from build123d import *

# Parameters (mm, degrees)
BOSS_EXTRUDE1_DEPTH                         = 300
CBORE_FOR_M3_BUTTON_HEAD_SCREW1_D           = 3.4
CBORE_FOR_M3_BUTTON_HEAD_SCREW1_CBORE_D     = 6.7
CBORE_FOR_M3_BUTTON_HEAD_SCREW1_CBORE_DEPTH = 6.15
LPATTERN1_COUNT                             = 12
LPATTERN1_PITCH                             = 25


with BuildPart() as part:
    # Sketch1 → Boss-Extrude1 (new body)
    with BuildSketch(Plane(origin=(0, 0, 0), x_dir=(0, 0, -1), z_dir=(1, 0, 0))):
        with BuildLine():
            Line((0, 5.5), (0, 0))
            Line((0, 0), (12, 0))
            Line((12, 0), (12, 5.5))
            ThreePointArc((12, 5.5), (11.5, 6), (12, 6.5))
            Line((12, 6.5), (12, 8))
            Line((12, 8), (0, 8))
            Line((0, 8), (0, 6.5))
            ThreePointArc((0, 6.5), (0.5, 6), (0, 5.5))
        make_face()
    extrude(amount=-BOSS_EXTRUDE1_DEPTH)

    # CBORE for M3 Button Head Screw1 (through all)
    with Locations(Plane(origin=(0, 8, 0), x_dir=(1, 0, 0), z_dir=(0, 1, 0))):
        with Locations((-288, 6)):
            cbore_for_m3_button_head_screw1 = CounterBoreHole(CBORE_FOR_M3_BUTTON_HEAD_SCREW1_D / 2, CBORE_FOR_M3_BUTTON_HEAD_SCREW1_CBORE_D / 2, CBORE_FOR_M3_BUTTON_HEAD_SCREW1_CBORE_DEPTH)

    # LPattern1: CBORE for M3 Button Head Screw1 ×12
    with Locations(*[(i * LPATTERN1_PITCH, 0, 0) for i in range(1, LPATTERN1_COUNT)]):
        add(cbore_for_m3_button_head_screw1, mode=Mode.SUBTRACT)


solid = part.part
The listing builds one solid part. Answer for the finished solid, in the listing's coordinates (mm). A direction names the side the tool comes from. Round coordinates to 2 decimals unless told otherwise and drop trailing zeros. Return JSON: item names as keys, results as strings.
Q1. Each of these flat-tipped pins is pushed along its axis until it touches: pin 1 Ø2.5 at (x, z) = (-188, -6) entering from -Y; pin 2 Ø2 at (x, z) = (-161.5, -6) entering from +Y. Where does it stop, or does it pass through?
Results list:
{"pin 1": "passes through", "pin 2": "stops at y = 1.85"}
Q2. Which of the six approach directions +Z, -Z, +X, -X, +Y, -Y give full straight-line access (tool end or side, diameter ignored) to faces 5 (the face through (-14, 1.85, -8)), 6 (the face through (-148, 3, 0))?
Results list:
{"face 5": "+Y", "face 6": "+Z, +X, -X, +Y, -Y"}
Q3. Find section A-A, the plane y = 3.25. State how many separate pieces and enclosed holes the cut face has, plus the area to 3 significant figures.
Results list:
{"separate pieces": "1", "enclosed holes": "12", "area": "3,180 mm2"}
Q4. Find the intervals of material crossed by line 1 along Z through (x, y) = (-213, 3.5); line 2 along Z through (x, y) = (-238, 1); line 3 along Y through (x, z) = (-263, -7.75), in increasing order. Write a range as from..to.
Results list:
{"line 1": "z = -12..-9.35, -2.65..0", "line 2": "z = -12..-7.7, -4.3..0", "line 3": "y = 0..1.85"}
Q5. The mould has two halves that part along X. Classify faces 1 (the face through (-148, 3, -12)), 2 (the face through (0, 4, -6)), 3 (the face through (-284.905, 4.968, -4.717)), 4 (the face through (-265, 1.85, -7)): released by +X, released by -X, zero draft, split by the parting line, or undercut.
Results list:
{"face 1": "zero draft", "face 2": "released by +X", "face 3": "undercut", "face 4": "undercut"}
